Verification items for this drawing (mm, ordinates from the low corner). A direction names the side the tool comes from. Round coordinates to 2 decimals unless told otherwise and drop trailing zeros. Loops run counter-clockwise (first coordinate to the right, second up) from the corner with the lowest first, then second, coordinate; pieces in that order, holes last. Notation, with made-up numbers: (-37, 1.5) -> (4, 1.5) arc R6 cw to (4, 8.5) -> close; hole circle Ø9 at (26.25, 77). An arc over 180 degrees is marked (long way). Use a Markdown table: item, result. Add a question column.
Q1. Sectioned sample at A-A, the plane x = 51. Enter the section's corners in (y, z).
Q2. Sectioned sample at B-B, the plane y = 11.5. Give the number of separate pieces and of enclosed holes in the cut face, then the cut area to 3 significant figures.
Q3. Release check for a two-part mould opening along Z. For the marked faces 4, 5 and 6 record: released by +Z, released by -Z, zero draft, split by the parting line, or undercut.
Q4. Sectioned sample at C-C, the plane x = 17. Enter the section's corners in (y, z).
Q5. Gauge pin test, flat ends, axial feed: P1, Ø1, axis at x = 12.5, z = 23.5, coming from the +Y side; P2, Ø3, axis at x = 17, z = 8.5, coming from the -Y side; P3, Ø2, axis at x = 21.5, y = 6.5, coming from the +Z side; P4, Ø19, axis at x = 44.5, y = 23.5, coming from the +Z side (1 decimal). Record the tip position at first contact, or that the pin passes through.
Q6. Material ranges on L1, parallel to Z at x = 51, y = 19; L2, parallel to X at y = 31, z = 34 (1 decimal); L3, parallel to Y at x = 4.5, z = 34, recorded low to high.
Q7. Sectioned sample at D-D, the plane z = 33.5. Enter the section's corners in (x, y) (1 decimal), then the cut area to 3 significant figures.
Q8. Set-up check for the marked faces 1, 2 and 3: record each of +Z, -Z, +X, -X, +Y, -Y from which the full face is reachable in a straight line by a thin tool's end or side.
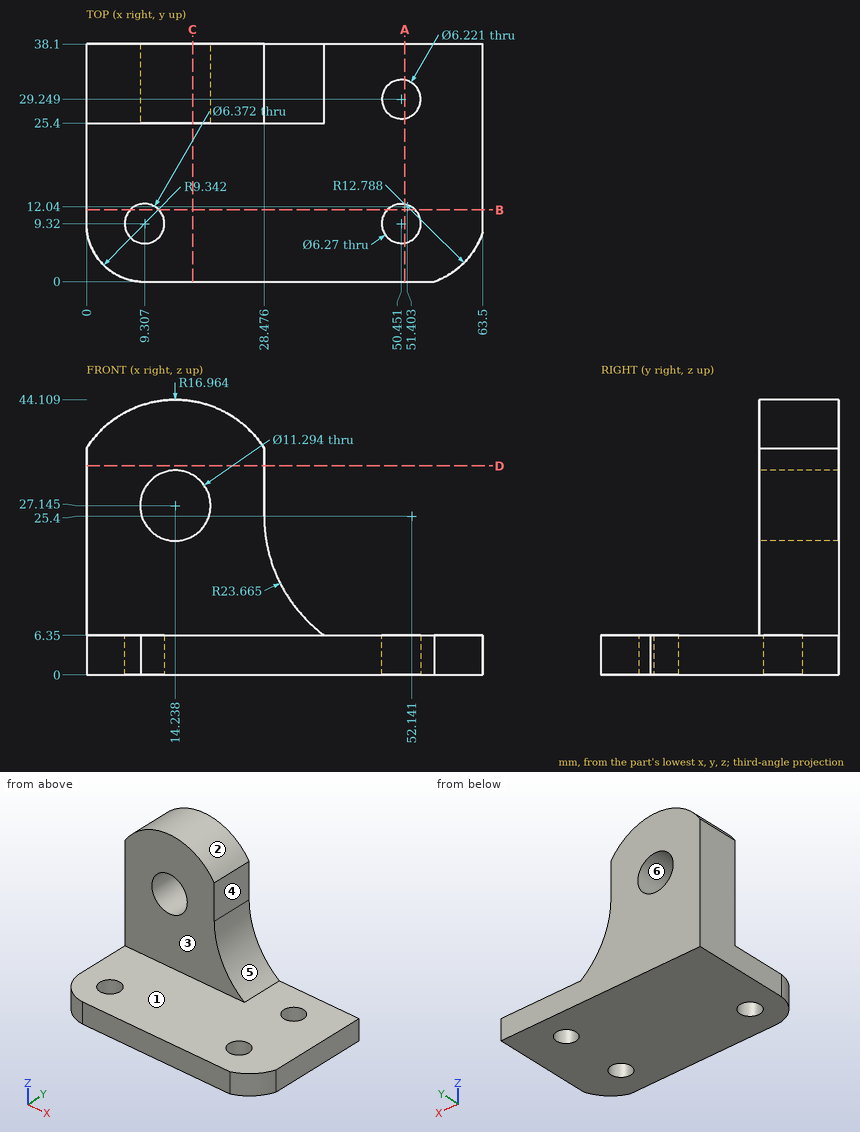
Values:
| question | item | result |
|---|---|---|
| 1 | outline | (0, 0) -> (6.23, 0) -> (6.23, 6.35) -> (0, 6.35) -> close; (12.41, 0) -> (26.19, 0) -> (26.19, 6.35) -> (12.41, 6.35) -> close; (32.31, 0) -> (38.1, 0) -> (38.1, 6.35) -> (32.31, 6.35) -> close |
| 2 | separate pieces | 3 |
| 2 | enclosed holes | 0 |
| 2 | area | 345 mm^2 |
| 3 | face 4 | zero draft |
| 3 | face 5 | released by +Z |
| 3 | face 6 | undercut |
| 4 | outline | (0, 0) -> (38.1, 0) -> (38.1, 22.22) -> (25.4, 22.22) -> (25.4, 6.35) -> (0, 6.35) -> close; (25.4, 32.07) -> (38.1, 32.07) -> (38.1, 43.88) -> (25.4, 43.88) -> close |
| 5 | P1 | through |
| 5 | P2 | y = 25.4 |
| 5 | P3 | z = 6.35 |
| 5 | P4 | z = 8.9 |
| 6 | L1 | 0 to 6.35 |
| 6 | L2 | 0 to 28.5 |
| 6 | L3 | 25.4 to 38.1 |
| 7 | outline | (0, 25.4) -> (28.5, 25.4) -> (28.5, 38.1) -> (0, 38.1) -> close |
| 7 | area | 362 mm^2 |
| 8 | face 1 | +Z, +X, -Y |
| 8 | face 2 | +Z, +Y, -Y |
| 8 | face 3 | +Z, +X, -X, -Y |
